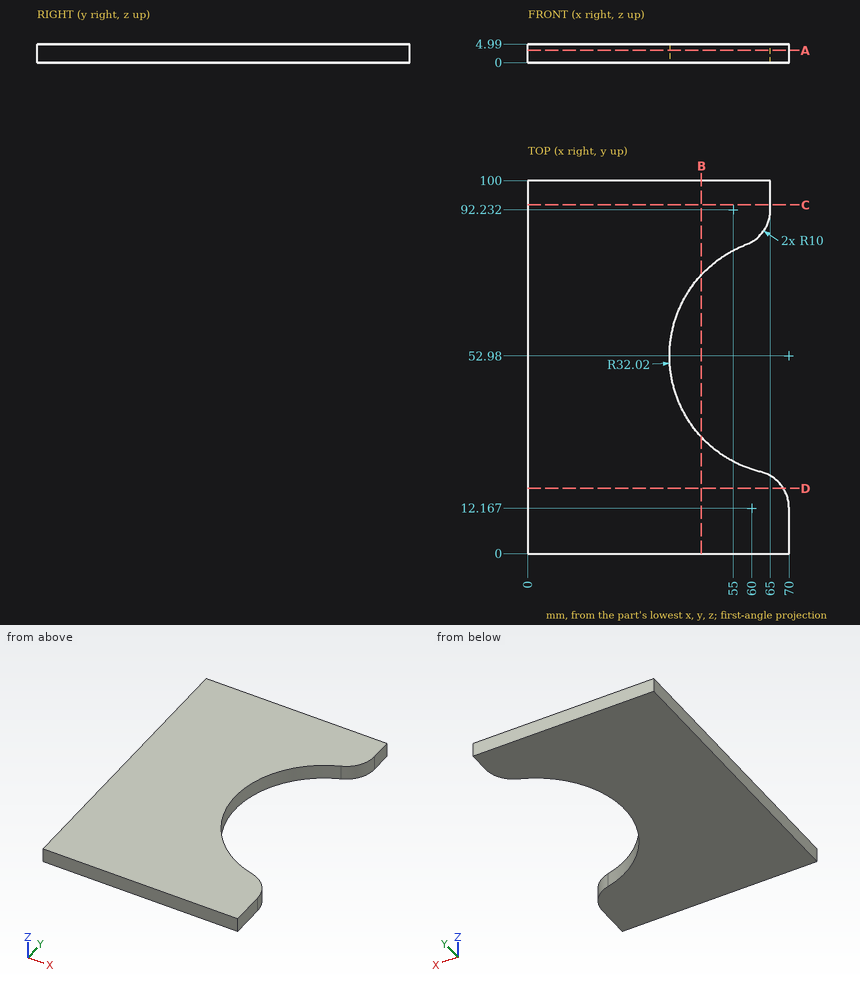
Study the drawing (mm; zero at the part's minimum x, y, z) and answer. Give positions to 0.01 mm unless a question says otherwise; leave off trailing zeros. Loops run counter-clockwise (first coordinate to the right, second up) from the corner with the lowest first, then second, coordinate; pieces in that order, holes last. Notation, with made-up numbers: M -20,5.5 L 30,5.5 A23 ccw 30,40.5 Z; hole C 47.5,-35.75 d4. An arc over 180 degrees is marked long. Answer as CSV lines item,"result".
Item 1: The part is cut by section D-D (y = 17.5). Give the vertices of the cut face in (x, z).
Values follow:
outline,"M 0,0 L 68.46,0 L 68.46,4.99 L 0,4.99 Z"
Item 2: The part is cut by section A-A (z = 3.25). Give the vertices of the cut face in (x, y), and give its area (3 significant figures).
Values follow:
outline,"M 0,0 L 70,0 L 70,12.17 A10 ccw 62.38,21.88 A32.02 cw 58.57,82.89 A10 ccw 65,92.23 L 65,100 L 0,100 Z"
area,"5,290 mm^2"
Item 3: The part is cut by section B-B (x = 46.5). Give the vertices of the cut face in (y, z), and give its area (3 significant figures).
Values follow:
outline,"M 0,0 L 31.23,0 L 31.23,4.99 L 0,4.99 Z; M 74.73,0 L 100,0 L 100,4.99 L 74.73,4.99 Z"
area,"282 mm^2"
Item 4: The part is cut by section C-C (y = 93.5). Give the vertices of the cut face in (x, z), and give its area (3 significant figures).
Values follow:
outline,"M 0,0 L 65,0 L 65,4.99 L 0,4.99 Z"
area,"324 mm^2"
Item 5: Straight lines are drawn through the part: line 1 along Y through (x, z) = (48.5, 4.25); line 2 along Y through (x, z) = (59, 3.6) (1 decimal); line 3 along X through (y, z) = (44.5, 1.9). For each, find the intervals that lie inside material, in ascending order. Write a range as [from, to].
Values follow:
line 1,"y = [0, 29.25], [76.71, 100]"
line 2,"y = [0, 22.9], [83.1, 100]"
line 3,"x = [0, 39.12]"
